from build123d import *
from build123d.topology import SkipClean

# Parameters (mm, degrees)
SKETCH2_W           = 240
SKETCH2_H           = 68
BOSS_EXTRUDE1_DEPTH = 15
SKETCH4_R           = 25
SKETCH4_R_2         = 15
BOSS_EXTRUDE4_DEPTH = 40
CUT_EXTRUDE2_START  = -40
SKETCH7_R           = 15
CUT_EXTRUDE2_DEPTH  = 40
BOSS_EXTRUDE5_DEPTH = 30
CUT_EXTRUDE3_DEPTH  = 77
RIB3_REACH          = 138.312
SKETCH11_WALL_W     = 307.624283584
SKETCH11_WALL_H     = 10
BOSS_EXTRUDE6_DEPTH = 8
SKETCH13_R          = 18
BOSS_EXTRUDE7_DEPTH = 42
SKETCH14_R          = 10
CUT_EXTRUDE4_DEPTH  = 67
RIB14_REACH         = 170.3
SKETCH19_WALL_W     = 410.192086974
SKETCH19_WALL_H     = 8


with BuildPart() as part:
    # Sketch2 → Boss-Extrude1 (new body)
    with BuildSketch(Plane(origin=(0, 0, 0), x_dir=(1, 0, 0), z_dir=(0, 1, 0))):
        Rectangle(SKETCH2_W, SKETCH2_H)
    extrude(amount=BOSS_EXTRUDE1_DEPTH)

    # Sketch4 → Boss-Extrude4 (add)
    with BuildSketch(Plane(origin=(0, 15, 0), x_dir=(1, 0, 0), z_dir=(0, 1, 0))):
        with Locations(Location((-82, 0, 0), (0, 0, 270))):
            Circle(SKETCH4_R)
        with Locations(Location((-82, 0, 0), (0, 0, 270))):
            Circle(SKETCH4_R_2, mode=Mode.SUBTRACT)
    extrude(amount=BOSS_EXTRUDE4_DEPTH)

    # Sketch7 → Cut-Extrude2 (cut)
    with BuildSketch(Plane(origin=(0, 15, 0), x_dir=(1, 0, 0), z_dir=(0, 1, 0)).offset(CUT_EXTRUDE2_START)):
        with Locations(Location((-82, 0, 0), (0, 0, 270))):
            Circle(SKETCH7_R)
    extrude(amount=CUT_EXTRUDE2_DEPTH, mode=Mode.SUBTRACT)

    # Sketch8 → Boss-Extrude5 (add)
    with BuildSketch(Plane(origin=(0, 15, 0), x_dir=(1, 0, 0), z_dir=(0, 1, 0))):
        with BuildLine():
            Line((-4, 20), (26, 20))
            ThreePointArc((26, 20), (46, 0), (26, -20))
            Line((26, -20), (-4, -20))
            ThreePointArc((-4, -20), (-24, 0), (-4, 20))
        make_face()
    extrude(amount=BOSS_EXTRUDE5_DEPTH)

    # Sketch9 → Cut-Extrude3 (cut)
    with BuildSketch(Plane(origin=(0, 45, 0), x_dir=(1, 0, 0), z_dir=(0, 1, 0))):
        with BuildLine():
            Line((-4, -10), (26, -10))
            ThreePointArc((26, -10), (36, 0), (26, 10))
            Line((26, 10), (-4, 10))
            ThreePointArc((-4, 10), (-14, 0), (-4, -10))
        make_face()
    extrude(amount=-CUT_EXTRUDE3_DEPTH, mode=Mode.SUBTRACT)

    # Sketch11 wall → Rib3 (add, up to next)
    with BuildSketch(Plane(origin=(-40.5, 35, 0), x_dir=(1, 0, 0), z_dir=(0, 1, 0)), mode=Mode.PRIVATE) as rib3_sk1:
        Rectangle(SKETCH11_WALL_W, SKETCH11_WALL_H)
    rib3_tool1 = extrude(rib3_sk1.sketch, amount=-RIB3_REACH, mode=Mode.PRIVATE) - part.part
    add(rib3_tool1.solids().sort_by_distance((-40.5, 35, 0))[0])

    # Sketch12 → Boss-Extrude6 (add)
    with BuildSketch(Plane(origin=(120, 0, 0), x_dir=(0, 0, -1), z_dir=(1, 0, 0))):
        with BuildLine():
            Line((-18, 95), (-34, 15))
            Line((-34, 15), (34, 15))
            Line((34, 15), (18, 95))
            ThreePointArc((18, 95), (0, 113), (-18, 95))
        make_face()
    extrude(amount=-BOSS_EXTRUDE6_DEPTH)

    # Sketch13 → Boss-Extrude7 (add)
    with SkipClean():  # the faces are left unmerged after this step: merging them gives an invalid solid
        with BuildSketch(Plane.ZY.offset(-112)):
            with Locations((0, 95)):
                Circle(SKETCH13_R)
        extrude(amount=BOSS_EXTRUDE7_DEPTH)
    add(part.part.scale(1), mode=Mode.REPLACE)  # the faces are merged on a copy

    # Sketch14 → Cut-Extrude4 (cut)
    with BuildSketch(Plane.ZY.offset(-70)):
        with Locations((0, 95)):
            Circle(SKETCH14_R)
    extrude(amount=-CUT_EXTRUDE4_DEPTH, mode=Mode.SUBTRACT)

    # Sketch19 wall → Rib14 (add, up to next)
    with BuildSketch(Plane(origin=(64.897858345, 46, 0), x_dir=(-0.500000000003, -0.866025403783, 0), z_dir=(0.866025403783, -0.500000000003, 0)), mode=Mode.PRIVATE) as rib14_sk1:
        Rectangle(SKETCH19_WALL_W, SKETCH19_WALL_H)
    rib14_tool1 = extrude(rib14_sk1.sketch, amount=RIB14_REACH, mode=Mode.PRIVATE) - part.part
    add(rib14_tool1.solids().sort_by_distance((64.897858345, 46, 0))[0])


solid = part.part
Model file for the job. Use its own axes, mm. A direction names the side the tool comes from. Coordinates: 2 decimals unless noted, no trailing zeros. Write each loop counter-clockwise with the first axis right and the second up, starting at its lowest first coordinate (ties: lowest second). Pieces come first, ordered by that corner, then holes. Notation, with made-up numbers: (48.5, 63.25) - (77.5, 63.25) arc R26 cw to (77.5, 85.25) - close; hole circle Ø2 at (61.25, 15). An arc over 180 degrees is marked (long way). Write each question's results on one line, items separated by ' | '. Start each with the question number.
1) Cut at A-A (x = 2). Write the cut outline in (y, z), then the cut area to 3 significant figures.
2) Cut at D-D (z = 29). Write the cut outline in (x, y), then the cut area to 3 significant figures.
3) Cut at C-C (x = -30). Write the cut outline in (y, z), then the cut area to 3 significant figures.
4) Flat gauge pins, fed straight in: P1, Ø16, axis at y = 95, z = 0, coming from the +X side; P2, Ø2, axis at x = 33.5, z = -12, coming from the +Y side; P3, Ø4, axis at x = -63, y = 29, coming from the -Z side; P4, Ø12, axis at y = 46.5, z = 10.5, coming from the -X side. Where does each tip first touch, or does it go through?
5) Cut at B-B (z = 0). Write the cut outline in (x, y), then the cut area to 3 significant figures.
6) Mould opens along Y. For faces 1 (the face through (65.3, 46.7, -0.1)), 2 (the face through (-93, 55, 11)), 3 (the face through (112, 47, -15)), 4 (the face through (46, 30, 0)) say: pulls with the +Y half, pulls with the -Y half, needs draft (parallel to the pull), parting line crosses it, or undercut.
7) 3-axis set-ups, long thin cutter, end or side, ignore diameter. For faces 5 (the face through (112, 47, 16)), 6 (the face through (-14, 23, 0)), 7 (the face through (11, 45, 13)), 8 (the face through (11, 30, 20)), 9 (the face through (-22.94, 29.79, -6.43)): which of +Z, -Z, +X, -X, +Y, -Y reach the whole face in a straight line?
8) Probe line 1 along Z through (x, y) = (-82, 19.5); line 2 along Z through (x, y) = (23.5, 19); line 3 along Y through (x, z) = (90, 0). List the from-to ranges inside material, lowest first. Write a range as from..to.
Returned:
1) outline: (0, -34) - (15, -34) - (15, -20) - (45, -20) - (45, -10) - (0, -10) - close; (0, 10) - (45, 10) - (45, 20) - (15, 20) - (15, 34) - (0, 34) - close | area: 1,320 mm^2
2) outline: (-120, 0) - (120, 0) - (120, 40) - (112, 40) - (112, 15) - (-120, 15) - close | area: 3,800 mm^2
3) outline: (0, -34) - (15, -34) - (15, -5) - (35, -5) - (35, 5) - (15, 5) - (15, 34) - (0, 34) - close | area: 1,220 mm^2
4) P1: through | P2: y = 45 | P3: z = -18.33 | P4: x = -106.59
5) outline: (-120, 0) - (-97, 0) - (-97, 55) - (-107, 55) - (-107, 15) - (-120, 15) - close; (-67, 0) - (-14, 0) - (-14, 45) - (-24, 45) - (-24, 35) - (-57, 35) - (-57, 55) - (-67, 55) - close; (36, 0) - (120, 0) - (120, 85) - (70, 85) - (70, 77) - (82.8, 77) - (47, 15) - (46, 15) - (46, 45) - (36, 45) - close; (70, 105) - (120, 105) - (120, 113) - (70, 113) - close | area: 8,680 mm^2
6) face 1: undercut | face 2: pulls with the +Y half | face 3: undercut | face 4: needs draft
7) face 5: +Z | face 6: +Y, -Y | face 7: +Z, -Z, +Y | face 8: +Z, +Y | face 9: +Y
8) line 1: -25..-15, 15..25 | line 2: -20..-10, 10..20 | line 3: 0..85, 105..113
